from build123d import *

# Parameters (mm, degrees)
SKETCH3_R           = 1.143
BOSS_EXTRUDE3_DEPTH = 3.81
CUT_EXTRUDE9_DEPTH  = 1.27
CUT_EXTRUDE10_DEPTH = 201.888951662
SKETCH11_W          = 43.18
SKETCH11_H          = 33.782
SKETCH11_R          = 3.81
SKETCH11_R_2        = 2.159
SKETCH11_R_3        = 6.985
CUT_EXTRUDE11_DEPTH = 201.888951662
CUT_EXTRUDE12_START = -1.27
SKETCH12_R          = 3.81
CUT_EXTRUDE12_DEPTH = 1.27
FILLET1_R           = 1.27


with BuildPart() as part:
    # Sketch3 → Boss-Extrude3 (new body)
    # profile 1 of 2: a face of its own
    with BuildSketch(Plane.XY):
        with BuildLine():
            Line((104.14, 0), (2.54, 0))
            ThreePointArc((2.54, 0), (0.743948776, -0.743948776), (0, -2.54))
            Line((0, -2.54), (0, -167.64))
            ThreePointArc((0, -167.64), (0.743948776, -169.436051224), (2.54, -170.18))
            Line((2.54, -170.18), (104.14, -170.18))
            ThreePointArc((104.14, -170.18), (105.936051224, -169.436051224), (106.68, -167.64))
            Line((106.68, -167.64), (106.68, -2.54))
            ThreePointArc((106.68, -2.54), (105.936051224, -0.743948776), (104.14, 0))
        make_face()
        with Locations(Location((101.6, -85.09, 0), (0, 0, 180))):
            Circle(SKETCH3_R, mode=Mode.SUBTRACT)
        with Locations(Location((5.08, -85.09, 0), (0, 0, 180))):
            Circle(SKETCH3_R, mode=Mode.SUBTRACT)
        with Locations(Location((5.08, -165.1, 0), (0, 0, 180))):
            Circle(SKETCH3_R, mode=Mode.SUBTRACT)
        with Locations(Location((101.6, -165.1, 0), (0, 0, 180))):
            Circle(SKETCH3_R, mode=Mode.SUBTRACT)
        with Locations(Location((5.08, -5.08, 0), (0, 0, 180))):
            Circle(SKETCH3_R, mode=Mode.SUBTRACT)
        with Locations(Location((101.6, -5.08, 0), (0, 0, 180))):
            Circle(SKETCH3_R, mode=Mode.SUBTRACT)
        with BuildLine():
            ThreePointArc((10.899871133, -2.54), (9.401860858, -3.199050905), (8.87556813, -4.748695652))
            ThreePointArc((8.87556813, -4.748695652), (7.774076836, -7.774076836), (4.748695652, -8.87556813))
            ThreePointArc((4.748695652, -8.87556813), (3.199050905, -9.401860858), (2.54, -10.899871133))
            Line((2.54, -10.899871133), (2.54, -79.270128867))
            ThreePointArc((2.54, -79.270128867), (3.199050905, -80.768139142), (4.748695652, -81.29443187))
            ThreePointArc((4.748695652, -81.29443187), (8.89, -85.09), (4.748695652, -88.88556813))
            ThreePointArc((4.748695652, -88.88556813), (3.199050905, -89.411860858), (2.54, -90.909871133))
            Line((2.54, -90.909871133), (2.54, -159.280128867))
            ThreePointArc((2.54, -159.280128867), (3.199050905, -160.778139142), (4.748695652, -161.30443187))
            ThreePointArc((4.748695652, -161.30443187), (7.774076836, -162.405923164), (8.87556813, -165.431304348))
            ThreePointArc((8.87556813, -165.431304348), (9.401860858, -166.980949095), (10.899871133, -167.64))
            Line((10.899871133, -167.64), (95.780128867, -167.64))
            ThreePointArc((95.780128867, -167.64), (97.278139142, -166.980949095), (97.80443187, -165.431304348))
            ThreePointArc((97.80443187, -165.431304348), (98.905923164, -162.405923164), (101.931304348, -161.30443187))
            ThreePointArc((101.931304348, -161.30443187), (103.480949095, -160.778139142), (104.14, -159.280128867))
            Line((104.14, -159.280128867), (104.14, -90.909871133))
            ThreePointArc((104.14, -90.909871133), (103.480949095, -89.411860858), (101.931304348, -88.88556813))
            ThreePointArc((101.931304348, -88.88556813), (97.79, -85.09), (101.931304348, -81.29443187))
            ThreePointArc((101.931304348, -81.29443187), (103.480949095, -80.768139142), (104.14, -79.270128867))
            Line((104.14, -79.270128867), (104.14, -10.899871133))
            ThreePointArc((104.14, -10.899871133), (103.480949095, -9.401860858), (101.931304348, -8.87556813))
            ThreePointArc((101.931304348, -8.87556813), (98.905923164, -7.774076836), (97.80443187, -4.748695652))
            ThreePointArc((97.80443187, -4.748695652), (97.278139142, -3.199050905), (95.780128867, -2.54))
            Line((95.780128867, -2.54), (10.899871133, -2.54))
        make_face(mode=Mode.SUBTRACT)
    # profile 2 of 2: a face of its own
    with BuildSketch(Plane.XY):
        with BuildLine():
            Line((10.899871133, -2.54), (95.780128867, -2.54))
            ThreePointArc((95.780128867, -2.54), (97.278139142, -3.199050905), (97.80443187, -4.748695652))
            ThreePointArc((97.80443187, -4.748695652), (98.905923164, -7.774076836), (101.931304348, -8.87556813))
            ThreePointArc((101.931304348, -8.87556813), (103.480949095, -9.401860858), (104.14, -10.899871133))
            Line((104.14, -10.899871133), (104.14, -79.270128867))
            ThreePointArc((104.14, -79.270128867), (103.480949095, -80.768139142), (101.931304348, -81.29443187))
            ThreePointArc((101.931304348, -81.29443187), (97.79, -85.09), (101.931304348, -88.88556813))
            ThreePointArc((101.931304348, -88.88556813), (103.480949095, -89.411860858), (104.14, -90.909871133))
            Line((104.14, -90.909871133), (104.14, -159.280128867))
            ThreePointArc((104.14, -159.280128867), (103.480949095, -160.778139142), (101.931304348, -161.30443187))
            ThreePointArc((101.931304348, -161.30443187), (98.905923164, -162.405923164), (97.80443187, -165.431304348))
            ThreePointArc((97.80443187, -165.431304348), (97.278139142, -166.980949095), (95.780128867, -167.64))
            Line((95.780128867, -167.64), (10.899871133, -167.64))
            ThreePointArc((10.899871133, -167.64), (9.401860858, -166.980949095), (8.87556813, -165.431304348))
            ThreePointArc((8.87556813, -165.431304348), (7.774076836, -162.405923164), (4.748695652, -161.30443187))
            ThreePointArc((4.748695652, -161.30443187), (3.199050905, -160.778139142), (2.54, -159.280128867))
            Line((2.54, -159.280128867), (2.54, -90.909871133))
            ThreePointArc((2.54, -90.909871133), (3.199050905, -89.411860858), (4.748695652, -88.88556813))
            ThreePointArc((4.748695652, -88.88556813), (8.89, -85.09), (4.748695652, -81.29443187))
            ThreePointArc((4.748695652, -81.29443187), (3.199050905, -80.768139142), (2.54, -79.270128867))
            Line((2.54, -79.270128867), (2.54, -10.899871133))
            ThreePointArc((2.54, -10.899871133), (3.199050905, -9.401860858), (4.748695652, -8.87556813))
            ThreePointArc((4.748695652, -8.87556813), (7.774076836, -7.774076836), (8.87556813, -4.748695652))
            ThreePointArc((8.87556813, -4.748695652), (9.401860858, -3.199050905), (10.899871133, -2.54))
        make_face()
    extrude(amount=BOSS_EXTRUDE3_DEPTH)

    # Sketch7 → Cut-Extrude9 (cut)
    with BuildSketch(Plane(origin=(0, 0, 0), x_dir=(-1, 0, 0), z_dir=(0, 0, -1))):
        with BuildLine():
            Line((-95.780128867, -2.54), (-10.899871133, -2.54))
            ThreePointArc((-10.899871133, -2.54), (-9.401860858, -3.199050905), (-8.87556813, -4.748695652))
            ThreePointArc((-8.87556813, -4.748695652), (-7.774076836, -7.774076836), (-4.748695652, -8.87556813))
            ThreePointArc((-4.748695652, -8.87556813), (-3.199050905, -9.401860858), (-2.54, -10.899871133))
            Line((-2.54, -10.899871133), (-2.54, -79.270128867))
            ThreePointArc((-2.54, -79.270128867), (-3.199050905, -80.768139142), (-4.748695652, -81.29443187))
            ThreePointArc((-4.748695652, -81.29443187), (-8.89, -85.09), (-4.748695652, -88.88556813))
            ThreePointArc((-4.748695652, -88.88556813), (-3.199050905, -89.411860858), (-2.54, -90.909871133))
            Line((-2.54, -90.909871133), (-2.54, -159.280128867))
            ThreePointArc((-2.54, -159.280128867), (-3.199050905, -160.778139142), (-4.748695652, -161.30443187))
            ThreePointArc((-4.748695652, -161.30443187), (-7.774076836, -162.405923164), (-8.87556813, -165.431304348))
            ThreePointArc((-8.87556813, -165.431304348), (-9.401860858, -166.980949095), (-10.899871133, -167.64))
            Line((-10.899871133, -167.64), (-95.780128867, -167.64))
            ThreePointArc((-95.780128867, -167.64), (-97.278139142, -166.980949095), (-97.80443187, -165.431304348))
            ThreePointArc((-97.80443187, -165.431304348), (-98.905923164, -162.405923164), (-101.931304348, -161.30443187))
            ThreePointArc((-101.931304348, -161.30443187), (-103.480949095, -160.778139142), (-104.14, -159.280128867))
            Line((-104.14, -159.280128867), (-104.14, -90.909871133))
            ThreePointArc((-104.14, -90.909871133), (-103.480949095, -89.411860858), (-101.931304348, -88.88556813))
            ThreePointArc((-101.931304348, -88.88556813), (-97.79, -85.09), (-101.931304348, -81.29443187))
            ThreePointArc((-101.931304348, -81.29443187), (-103.480949095, -80.768139142), (-104.14, -79.270128867))
            Line((-104.14, -79.270128867), (-104.14, -36.557585396))
            Line((-104.14, -36.557585396), (-104.14, -10.899871133))
            ThreePointArc((-104.14, -10.899871133), (-103.480949095, -9.401860858), (-101.931304348, -8.87556813))
            ThreePointArc((-101.931304348, -8.87556813), (-98.905923164, -7.774076836), (-97.80443187, -4.748695652))
            ThreePointArc((-97.80443187, -4.748695652), (-97.278139142, -3.199050905), (-95.780128867, -2.54))
        make_face()
    extrude(amount=-CUT_EXTRUDE9_DEPTH, mode=Mode.SUBTRACT)

    # Sketch10 → Cut-Extrude10 (cut, through all)
    with BuildSketch(Plane.XY.offset(3.81)):
        Polygon((2.54, -21.336), (0, -21.336), (0, -36.576), (2.54, -36.576), (5.08, -36.576), (5.08, -21.336), align=None)
    extrude(amount=-CUT_EXTRUDE10_DEPTH, mode=Mode.SUBTRACT)

    # Sketch11 → Cut-Extrude11 (cut, through all)
    with BuildSketch(Plane.XY.offset(3.81)):
        with Locations((45.212, -37.211)):
            Rectangle(SKETCH11_W, SKETCH11_H)
        with Locations((10.668, -45.72)):
            Circle(SKETCH11_R)
        with Locations((26.7462, -59.69)):
            Circle(SKETCH11_R_2)
        with Locations((91.44, -35.56)):
            Circle(SKETCH11_R_3)
    extrude(amount=-CUT_EXTRUDE11_DEPTH, mode=Mode.SUBTRACT)

    # Sketch12 → Cut-Extrude12 (cut)
    with BuildSketch(Plane.XY.offset(3.81).offset(CUT_EXTRUDE12_START)):
        with Locations((5.08, -5.08)):
            Circle(SKETCH12_R)
        with Locations((101.6, -5.08)):
            Circle(SKETCH12_R)
        with Locations((101.6, -85.09)):
            Circle(SKETCH12_R)
        with Locations((101.6, -165.1)):
            Circle(SKETCH12_R)
        with Locations((5.08, -165.1)):
            Circle(SKETCH12_R)
        with Locations((5.08, -85.09)):
            Circle(SKETCH12_R)
    extrude(amount=CUT_EXTRUDE12_DEPTH, mode=Mode.SUBTRACT)

    # Fillet1
    fillet1_edges = [part.edges().sort_by_distance(p)[0] for p in [
        (0, -102.108, 3.81),
        (5.08, -28.956, 3.81),
        (2.54, -36.576, 3.81),
        (2.54, -21.336, 3.81),
        (53.34, 0, 3.81),
        (0.743948776, -0.743948776, 3.81),
        (0, -11.938, 3.81),
        (0.743948776, -169.436051224, 3.81),
        (53.34, -170.18, 3.81),
        (105.936051224, -169.436051224, 3.81),
        (106.68, -85.09, 3.81),
        (105.936051224, -0.743948776, 3.81),
    ]]
    fillet(fillet1_edges, radius=FILLET1_R - 0.0001)  # a hair under: the kernel refuses the full size


solid = part.part
Read the model definition and answer for the solid it produces. Units are mm, in the model's axes. A direction names the side the tool comes from. Give positions to 0.01 mm unless a question says otherwise; leave off trailing zeros. Write each loop counter-clockwise with the first axis right and the second up, starting at its lowest first coordinate (ties: lowest second). Pieces come first, ordered by that corner, then holes. Notation, with made-up numbers: M 89.25,75 L 111.25,75 A24 ccw 111.25,89 Z; hole C 58.5,18 d5. An arc over 180 degrees is marked long. One line per item, written item: value. Start each with the question number.
(1) Find section A-A (y = -59.69). Determine the outline of the cut face in (x, z).
(2) A tool of negligible diameter and unlimited length cuts with its end or side. For faces 1 (the cylindrical face through (14.302, -44.576, 2.558)), 2 (the flat face through (102, -7, 2.54)), 3 (the cylindrical face through (98.87, -162.44, 0.63)), from which of +Z, -Z, +X, -X, +Y, -Y can it reach the whole face along a straight path? Write none if from no direction.
(3) Find section D-D (x = 17.5). Determine the outline of the cut face in (y, z).
(4) Find the intervals of material crossed by line 1 (Y direction, x = 5.08, z = 0.95); line 2 (Y direction, x = 96, z = 1.1); line 3 (Y direction, x = 5.08, z = 3.3), in increasing order.
(5) Find section B-B (x = 91.44). Determine the outline of the cut face in (y, z) (3 decimals), plus the area to 3 significant figures.
(6) Flat-ended cylindrical pins translate along their axes: pin 1 Ø7 at (x, y) = (5.08, -85.09) entering from -Z; pin 2 Ø1.4 at (x, y) = (101.6, -85.09) entering from -Z; pin 3 Ø4 at (x, y) = (102, -85) entering from +Z; pin 4 Ø1.3 at (x, z) = (1.5, 2) entering from +Y. Find the tip coordinate at first contact, or state that the pin passes through.
(7) Determine the mould class of faces 4 (the flat face through (105, -85, 0)), 5 (the cylindrical face through (98.94, -7.81, 0.63)) for opening direction Y: pulls with the +Y half, pulls with the -Y half, needs draft (parallel to the pull), parting line crosses it, or undercut.
(8) Find section C-C (y = -111). Determine the outline of the cut face in (x, z).
Results below:
1. outline: M 0,0 L 2.54,0 L 2.54,1.27 L 24.59,1.27 L 24.59,3.81 L 1.27,3.81 A1.27 ccw 0,2.54 Z; M 28.91,1.27 L 104.14,1.27 L 104.14,0 L 106.68,0 L 106.68,2.54 A1.27 ccw 105.41,3.81 L 28.91,3.81 Z
2. face 1: +Z, -Z
2. face 2: +Z
2. face 3: -Z
3. outline: M -170.18,0 L -167.64,0 L -167.64,1.27 L -2.54,1.27 L -2.54,0 L 0,0 L 0,2.54 A1.27 ccw -1.27,3.81 L -168.91,3.81 A1.27 ccw -170.18,2.54 Z
4. line 1: y = -170.18 to -166.24, -163.96 to -161.29, -88.9 to -86.23, -83.95 to -81.28, -8.89 to -6.22, -3.94 to 0
4. line 2: y = -170.18 to -167.63, -2.55 to 0
4. line 3: y = -169.93 to -168.91, -161.29 to -88.9, -81.28 to -36.83, -21.08 to -8.89, -1.27 to -0.25
5. outline: M -170.18,0 L -167.64,0 L -167.64,1.27 L -42.545,1.27 L -42.545,3.81 L -168.91,3.81 A1.27 ccw -170.18,2.54 Z; M -28.575,1.27 L -2.54,1.27 L -2.54,0 L 0,0 L 0,2.54 A1.27 ccw -1.27,3.81 L -28.575,3.81 Z
5. area: 403 mm^2
6. pin 1: stops at z = 0
6. pin 2: passes through
6. pin 3: stops at z = 2.54
6. pin 4: stops at y = -0.03
7. face 4: needs draft
7. face 5: undercut
8. outline: M 0,0 L 2.54,0 L 2.54,1.27 L 104.14,1.27 L 104.14,0 L 106.68,0 L 106.68,2.54 A1.27 ccw 105.41,3.81 L 1.27,3.81 A1.27 ccw 0,2.54 Z
